Design review of the part built by this model. Coordinates are the model's own, in mm. A direction names the side the tool comes from. Round coordinates to 2 decimals unless told otherwise and drop trailing zeros. Order: outer loops, then holes, each group sorted by start corner. A loop starts at its lowest first (then second) coordinate and runs counter-clockwise, first axis right, second up. Notation, with made-up numbers: M 53,44 L 63,44 A21 cw 63,66 Z; hole C -4.75,65.5 d1. An arc over 180 degrees is marked long. Use a Markdown table: item, result. Add a question column.
(1) For pin 1 (10 mm diameter, centred on x = 91.5, y = -19.5, fed in from +Z); pin 2 (10 mm diameter, centred on x = 2.5, z = -1.5, fed in from -Y); pin 3 (1.6 mm diameter, centred on y = -22.5, z = -99, fed in from +X), all flat-tipped, find the tip position at first contact; note any pin that passes through.
(2) Take a section at A-A (y = -50.5). Write out the cut boundary in (x, z), then the cut area to 3 significant figures.
(3) Take a section at C-C (x = -19.5). Write out the cut boundary in (y, z).
(4) To check wall thickness, follow probe 1 along Z at (x, y) = (-84.6, -32.12); probe 2 along Z at (x, y) = (-43.5, -47); probe 3 along Y at (x, z) = (11, 36). State the ranges of each line that lie inside material, in increasing order. Write a range as from..to.
(5) The part is to be moulded in two halves that separate along Z. For faces 1 (the face through (-47, -31, -100)), 2 (the face through (88, -19, -50)), 3 (the face through (-4, 0, -19)), say which applies: released by +Z, released by -Z, zero draft, split by the parting line, or undercut.
(6) Take a section at B-B (z = -42.5). Write out the cut boundary in (x, y), then the cut area to 3 significant figures.
(7) Machinability: for faces 4 (the face through (-84.3, -31.79, -83.63)), 5 (the face through (93.524, -29.92, -21.05)), 6 (the face through (-46, -32, 58)), which of the approach directions +Z, -Z, +X, -X, +Y, -Y give a long, thin tool a straight path to every point of the face, cutting with its end or side? Answer none if there is none.
(8) Take a section at D-D (z = 40). Write out the cut boundary in (x, y), then the cut area to 3 significant figures.
```python
from build123d import *

# Parameters (mm, degrees)
SKETCH1_W                    = 160
SKETCH1_H                    = 150
BASE_FLANGE1_DEPTH           = 2
EDGE_FLANGE1_START           = -95
EDGE_FLANGE1_DEPTH           = 150
EDGE_FLANGE2_STRIP_W         = 20
EDGE_FLANGE2_STRIP_H         = 2
EDGE_FLANGE2_STRIP_CUT_DEPTH = 150
EDGE_FLANGE2_DEPTH           = 150
EDGE_FLANGE4_DEPTH           = 159.113248654
EDGE_FLANGE5_DEPTH           = 159.113248654
SKETCH32_W                   = 30
SKETCH32_H                   = 21.454922416
CUT_EXTRUDE2_DEPTH           = 10
SKETCH33_W                   = 87.917980444
SKETCH33_H                   = 57
CUT_EXTRUDE3_DEPTH           = 199.782165551
SKETCH38_R                   = 2.5
CUT_EXTRUDE5_DEPTH           = 2
SKETCH39_R                   = 2.5
CUT_EXTRUDE6_DEPTH           = 3


# Read off the part's stored shape, not the designer's step: Edge-Flange1
# Sheet-metal steps are written as plain solids
with BuildPart() as part:
    # Sketch1 → Base-Flange1 (new body)
    with BuildSketch(Plane(origin=(0, 0, 0), x_dir=(1, 0, 0), z_dir=(0, 1, 0))):
        with Locations((-5.285714286, 20)):
            Rectangle(SKETCH1_W, SKETCH1_H)
    extrude(amount=-BASE_FLANGE1_DEPTH)

    # Edge-Flange1 outline → Edge-Flange1 (add)
    with BuildSketch(Plane.XY.offset(EDGE_FLANGE1_START)):
        with BuildLine():
            Line((101.559585176, -39.837168574), (79.42561058, -1.5))
            ThreePointArc((79.42561058, -1.5), (78.327534368, -0.401923789), (76.827534368, 0))
            Line((76.827534368, 0), (74.714285714, 0))
            Line((74.714285714, 0), (74.714285714, -2))
            Line((74.714285714, -2), (76.827534368, -2))
            ThreePointArc((76.827534368, -2), (77.327534368, -2.133974596), (77.693559772, -2.5))
            Line((77.693559772, -2.5), (99.827534368, -40.837168574))
            Line((99.827534368, -40.837168574), (101.559585176, -39.837168574))
        make_face()
    extrude(amount=EDGE_FLANGE1_DEPTH)

    # Edge-Flange2 strip (across the edge) → Edge-Flange2 strip cut (cut)
    with BuildSketch(Plane(origin=(-85.285714286, -2, 55), x_dir=(1, 0, 0), z_dir=(0, 0, -1))):
        with Locations((-7, -1)):
            Rectangle(EDGE_FLANGE2_STRIP_W, EDGE_FLANGE2_STRIP_H)
    extrude(amount=EDGE_FLANGE2_STRIP_CUT_DEPTH, mode=Mode.SUBTRACT)

    # Edge-Flange2 section (across the edge) → Edge-Flange2 (add)
    with BuildSketch(Plane(origin=(-85.285714286, -2, 55), x_dir=(1, 0, 0), z_dir=(0, 0, -1))):
        with BuildLine():
            Line((0, 1), (0, 38))
            Line((0, 38), (2, 38))
            Line((2, 38), (2, 1))
            ThreePointArc((2, 1), (2.292893219, 0.292893219), (3, 0))
            Line((3, 0), (3, -2))
            ThreePointArc((3, -2), (0.878679656, -1.121320344), (0, 1))
        make_face()
    extrude(amount=EDGE_FLANGE2_DEPTH)

    # Edge-Flange4 section (across the edge) → Edge-Flange4 (add)
    with BuildSketch(Plane(origin=(76.827534368, -2, 60), x_dir=(0, 0, -1), z_dir=(-1, 0, 0))):
        with BuildLine():
            Line((0, 1), (0, 58))
            Line((0, 58), (2, 58))
            Line((2, 58), (2, 1))
            ThreePointArc((2, 1), (2.292893219, 0.292893219), (3, 0))
            Line((3, 0), (5, 0))
            Line((5, 0), (5, -2))
            Line((5, -2), (3, -2))
            ThreePointArc((3, -2), (0.878679656, -1.121320344), (0, 1))
        make_face()
    extrude(amount=EDGE_FLANGE4_DEPTH)

    # Edge-Flange5 section (across the edge) → Edge-Flange5 (add)
    with BuildSketch(Plane(origin=(-82.285714286, -2, -100), x_dir=(0, 0, 1), z_dir=(1, 0, 0))):
        with BuildLine():
            Line((0, 1), (0, 58))
            Line((0, 58), (2, 58))
            Line((2, 58), (2, 1))
            ThreePointArc((2, 1), (2.292893219, 0.292893219), (3, 0))
            Line((3, 0), (5, 0))
            Line((5, 0), (5, -2))
            Line((5, -2), (3, -2))
            ThreePointArc((3, -2), (0.878679656, -1.121320344), (0, 1))
        make_face()
    extrude(amount=EDGE_FLANGE5_DEPTH)

    # Sketch32 → Cut-Extrude2 (cut)
    with BuildSketch(Plane(origin=(58.919688882, 34.017298237, 0), x_dir=(0, 0, -1), z_dir=(0.8660254037844364, 0.5000000000000039, 0))):
        with Locations((5, -60.695720616)):
            Rectangle(SKETCH32_W, SKETCH32_H)
        with Locations((35, -60.695720616)):
            Rectangle(SKETCH32_W, SKETCH32_H)
    extrude(amount=-CUT_EXTRUDE2_DEPTH, mode=Mode.SUBTRACT)

    # Sketch33 → Cut-Extrude3 (cut, through all)
    with BuildSketch(Plane.XY.offset(60)):
        with Locations((32.868544146, -31.5)):
            Rectangle(SKETCH33_W, SKETCH33_H)
    extrude(amount=-CUT_EXTRUDE3_DEPTH, mode=Mode.SUBTRACT)

    # Sketch38 → Cut-Extrude5 (cut)
    with BuildSketch(Plane(origin=(58.919688882, 34.017298237, 0), x_dir=(0, 0, -1), z_dir=(0.8660254037844363, 0.5000000000000042, 0))):
        with Locations(Location((-46, -78, 0), (0, 0, 90))):
            Circle(SKETCH38_R)
        with Locations(Location((86, -78, 0), (0, 0, 270))):
            Circle(SKETCH38_R)
    extrude(amount=-CUT_EXTRUDE5_DEPTH, mode=Mode.SUBTRACT)

    # Sketch39 → Cut-Extrude6 (cut)
    with BuildSketch(Plane.ZY.offset(85.285714286)):
        with Locations(Location((46.11, -32.12, 0), (0, 0, 270))):
            Circle(SKETCH39_R)
        with Locations(Location((-86.11, -32.12, 0), (0, 0, 270))):
            Circle(SKETCH39_R)
    extrude(amount=-CUT_EXTRUDE6_DEPTH, mode=Mode.SUBTRACT)


solid = part.part
```
Verdict:
| question | item | result |
|---|---|---|
| 1 | pin 1 | stops at z = 55 |
| 1 | pin 2 | stops at y = -2 |
| 1 | pin 3 | stops at x = -11.09 |
| 2 | outline | M -82.29,-100 L -11.09,-100 L -11.09,-98 L -82.29,-98 Z; M -82.29,58 L -11.09,58 L -11.09,60 L -82.29,60 Z |
| 2 | area | 285 mm^2 |
| 3 | outline | M -60,-100 L -3,-100 A3 ccw 0,-97 L 0,57 A3 ccw -3,60 L -60,60 L -60,58 L -3,58 A1 cw -2,57 L -2,-97 A1 cw -3,-98 L -60,-98 Z |
| 4 | probe 1 | z = -95..-88.61, -83.61..43.61, 48.61..55 |
| 4 | probe 2 | z = -100..-98, 58..60 |
| 4 | probe 3 | y = -2..0 |
| 5 | face 1 | released by -Z |
| 5 | face 2 | undercut |
| 5 | face 3 | zero draft |
| 6 | outline | M -85.29,-40 L -83.29,-40 L -83.29,-3 A1 cw -82.29,-2 L 76.83,-2 A1 cw 77.69,-2.5 L 82.17,-10.26 L 83.9,-9.26 L 79.43,-1.5 A3 ccw 76.83,0 L -82.29,0 A3 ccw -85.29,-3 Z; M 92.9,-28.84 L 99.83,-40.84 L 101.56,-39.84 L 94.63,-27.84 Z |
| 6 | area | 448 mm^2 |
| 7 | face 4 | -X |
| 7 | face 5 | +Z, -Z, -Y |
| 7 | face 6 | +X, -X, -Y |
| 8 | outline | M -85.29,-40 L -83.29,-40 L -83.29,-3 A1 cw -82.29,-2 L 76.83,-2 A1 cw 77.69,-2.5 L 99.83,-40.84 L 101.56,-39.84 L 79.43,-1.5 A3 ccw 76.83,0 L -82.29,0 A3 ccw -85.29,-3 Z |
| 8 | area | 491 mm^2 |
